For this review, take the finished solid that the model builds, in its own axes (mm). Round coordinates to 2 decimals unless told otherwise and drop trailing zeros. Order: outer loops, then holes, each group sorted by start corner. A loop starts at its lowest first (then second) coordinate and runs counter-clockwise, first axis right, second up. Notation, with made-up numbers: (45, 40) - (50, 40) arc R21 cw to (50, 55) - close; hole circle Ø6 at (69.25, 75). An arc over 180 degrees is marked (long way). Write each question's results on one line, items separated by ' | '. Start each with the question number.
(1) Take a section at A-A, the plane z = 13.25. Give the boundary of the cut face in (x, y), plus the area to 3 significant figures.
(2) Insertion check: pin 1 Ø5 at (y, z) = (8.5, 6) entering from +X; pin 2 Ø4 at (x, y) = (62.5, 30.5) entering from -Z; pin 3 Ø8 at (y, z) = (13.5, 17.5) entering from -X; pin 4 Ø1 at (x, z) = (61, 11) entering from +Y. Each pin has a flat end and moves straight along its axis. Give the tip position at first contact, or say it passes through.
(3) For L1, parallel to X at y = 7.5, z = 11.75; L2, parallel to X at y = 27.5, z = 2, list the stretches that pass through material, from the lowest coordinate up. Write a range as from..to.
(4) Take a section at B-B, the plane y = 12.5. Give the boundary of the cut face in (x, z).
(5) Draft analysis for pull direction Y (two halves, no side actions). For faces 1 (the flat face through (64, 23, 0)), 2 (the flat face through (64.31, 22.92, 9.86)), 3 (the cylindrical face through (59.97, 40.52, 8.57)), state which applies: pulls with the +Y half, pulls with the -Y half, needs draft (parallel to the pull), parting line crosses it, or undercut.
Autodesk Inventor part; units mm, degrees
ref_plane "YZ Plane" through (0, 0, 0) normal (1, 0, 0) x (0, 1, 0)
ref_plane "XZ Plane" through (0, 0, 0) normal (0, 1, 0) x (-1, 0, 0)
ref_plane "XY Plane" through (0, 0, 0) normal (0, 0, 1) x (1, 0, 0)
sketch "スケッチ1" plane through (0, 0, 0) normal (0, 0, 1) x (1, 0, 0)
  circle A0 centre (54.6996, 44) radius 4
  line L0 (61.9927, 0) -> (64.9927, 0)
  line L1 (58.602, 44.878) -> (68.6996, 0)
  line L2 (64.9927, 0) -> (67.602, 4.878)
  line L3 (59.3337, 45.0427) -> (69.4313, 0.1646)
  line L4 (59.3337, 45.0427) -> (58.602, 44.878)
  line L5 (68.6996, 0) -> (69.4313, 0.1646)
  point P0 (0, 0)
  dimension "d0" = 5
  dimension "d1" = 0.75
  dimension "d12" = 77.32
extrude "押し出し1" add sketch "スケッチ1" along normal blind 20 contours L4 L3 L5 L1
sketch "スケッチ2" plane through (59.3337, 45.0427, 20) normal (0.9756, 0.2195, 0) x (0, 0, -1)
  line L0 (20, -46) -> (20, 0)
  line L1 (20, 0) -> (0, 0)
  line L2 (0, -46) -> (0, 0)
  line L3 (20, -46) -> (0, -46)
  circle A0 centre (10, -41) radius 1.5
  circle A1 centre (10, -5) radius 1.5
  point P0 (20, -30.9196)
  dimension "d4" = 3
  dimension "d5" = 5
  dimension "d6" = 10
  dimension "d7" = 3
  dimension "d8" = 5
  dimension "d9" = 10
extrude "押し出し2" cut sketch "スケッチ2" against normal blind 0.75 contours A0 | A1
properties part number "アームガード" material "ポリプロピレン"
Results below:
1) outline: (58.6, 44.88) - (68.7, 0) - (69.43, 0.16) - (59.33, 45.04) - close | area: 34.5 mm^2
2) pin 1: stops at x = 68.12 | pin 2: stops at z = 0 | pin 3: stops at x = 64.76 | pin 4: stops at y = 39.43
3) L1: x = 67.01..67.78 | L2: x = 62.51..63.28
4) outline: (65.89, 0) - (66.66, 0) - (66.66, 20) - (65.89, 20) - close
5) face 1: needs draft | face 2: pulls with the +Y half | face 3: undercut
